from build123d import *

# Parameters (mm, degrees)
SALIENTE_EXTRUIR1_DEPTH = 35
CORTAR_EXTRUIR1_REACH   = 64.883
CROQUIS2_R              = 2.55
CROQUIS3_R              = 4.75
CORTAR_EXTRUIR2_DEPTH   = 17
CHAFL_N1_SIZE           = 15
CHAFL_N1_SIZE_2         = 21.422220101
CORTAR_EXTRUIR3_START   = -35
CROQUIS4_W              = 81
CROQUIS4_H              = 1
CORTAR_EXTRUIR3_DEPTH   = 35


with BuildPart() as part:
    # Croquis1 → Saliente-Extruir1 (new body)
    with BuildSketch(Plane(origin=(0, 0, 0), x_dir=(1, 0, 0), z_dir=(0, 1, 0))):
        with BuildLine():
            Line((22.5, 0), (40.5, 0))
            Line((40.5, 0), (40.5, -33))
            Line((40.5, -33), (-40.5, -33))
            Line((-40.5, -33), (-40.5, 0))
            Line((-40.5, 0), (-22.5, 0))
            ThreePointArc((-22.5, 0), (0, -22.5), (22.5, 0))
        make_face()
    extrude(amount=SALIENTE_EXTRUIR1_DEPTH)

    # Croquis2 → Cortar-Extruir1 (cut, up to next)
    with BuildSketch(Plane(origin=(0, 0, 0), x_dir=(-1, 0, 0), z_dir=(0, 0, -1)), mode=Mode.PRIVATE) as cortar_extruir1_sk1:
        with Locations((-31.5, 26.25)):
            Circle(CROQUIS2_R)
    cortar_extruir1_tool1 = extrude(cortar_extruir1_sk1.sketch, amount=-CORTAR_EXTRUIR1_REACH, mode=Mode.PRIVATE) & part.part
    # Croquis2 → Cortar-Extruir1 (cut, up to next)
    with BuildSketch(Plane(origin=(0, 0, 0), x_dir=(-1, 0, 0), z_dir=(0, 0, -1)), mode=Mode.PRIVATE) as cortar_extruir1_sk2:
        with Locations((-31.5, 8.75)):
            Circle(CROQUIS2_R)
    cortar_extruir1_tool2 = extrude(cortar_extruir1_sk2.sketch, amount=-CORTAR_EXTRUIR1_REACH, mode=Mode.PRIVATE) & part.part
    # Croquis2 → Cortar-Extruir1 (cut, up to next)
    with BuildSketch(Plane(origin=(0, 0, 0), x_dir=(-1, 0, 0), z_dir=(0, 0, -1)), mode=Mode.PRIVATE) as cortar_extruir1_sk3:
        with Locations((31.5, 8.75)):
            Circle(CROQUIS2_R)
    cortar_extruir1_tool3 = extrude(cortar_extruir1_sk3.sketch, amount=-CORTAR_EXTRUIR1_REACH, mode=Mode.PRIVATE) & part.part
    # Croquis2 → Cortar-Extruir1 (cut, up to next)
    with BuildSketch(Plane(origin=(0, 0, 0), x_dir=(-1, 0, 0), z_dir=(0, 0, -1)), mode=Mode.PRIVATE) as cortar_extruir1_sk4:
        with Locations((31.5, 26.25)):
            Circle(CROQUIS2_R)
    cortar_extruir1_tool4 = extrude(cortar_extruir1_sk4.sketch, amount=-CORTAR_EXTRUIR1_REACH, mode=Mode.PRIVATE) & part.part
    add(cortar_extruir1_tool1.solids().sort_by_distance((31.5, 26.25, 0))[0], mode=Mode.SUBTRACT)
    add(cortar_extruir1_tool2.solids().sort_by_distance((31.5, 8.75, 0))[0], mode=Mode.SUBTRACT)
    add(cortar_extruir1_tool3.solids().sort_by_distance((-31.5, 8.75, 0))[0], mode=Mode.SUBTRACT)
    add(cortar_extruir1_tool4.solids().sort_by_distance((-31.5, 26.25, 0))[0], mode=Mode.SUBTRACT)

    # Croquis3 → Cortar-Extruir2 (cut)
    with BuildSketch(Plane.XY.offset(33)):
        with Locations((-31.5, 26.25)):
            Circle(CROQUIS3_R)
        with Locations((-31.5, 8.75)):
            Circle(CROQUIS3_R)
        with Locations((31.5, 26.25)):
            Circle(CROQUIS3_R)
        with Locations((31.5, 8.75)):
            Circle(CROQUIS3_R)
    extrude(amount=-CORTAR_EXTRUIR2_DEPTH, mode=Mode.SUBTRACT)

    # Chaflán1
    # the kernel refuses this chamfer: 21.422220101, 15 mm, written as the material it takes off along each edge
    with BuildSketch(Plane(origin=(40.5, -55.3240023, 33), x_dir=(0.045263737714021264, 0, -0.9989750717851553), z_dir=(0, 1, 0))) as chafl_n1_piece_1:
        Polygon((CHAFL_N1_SIZE * 0.998975071785, CHAFL_N1_SIZE * 0.045263737714), (-CHAFL_N1_SIZE_2 * 0.0452637377143, CHAFL_N1_SIZE_2 * 0.998975071791), (0, 0), align=None)
    extrude(amount=145.6480046, mode=Mode.SUBTRACT)
    with BuildSketch(Plane(origin=(-40.5, -55.3240023, 33), x_dir=(0.9997533347641299, 0, 0.022209674198456895), z_dir=(0, 1, 0))) as chafl_n1_piece_2:
        Polygon((CHAFL_N1_SIZE_2 * 0.99975333477, CHAFL_N1_SIZE_2 * 0.0222096741986), (-CHAFL_N1_SIZE * 0.0222096741985, CHAFL_N1_SIZE * 0.999753334764), (0, 0), align=None)
    extrude(amount=145.6480046, mode=Mode.SUBTRACT)

    # Croquis4 → Cortar-Extruir3 (cut)
    with BuildSketch(Plane(origin=(0, 35, 0), x_dir=(1, 0, 0), z_dir=(0, 1, 0)).offset(CORTAR_EXTRUIR3_START)):
        with Locations((0, -0.5)):
            Rectangle(CROQUIS4_W, CROQUIS4_H)
    extrude(amount=CORTAR_EXTRUIR3_DEPTH, mode=Mode.SUBTRACT)


solid = part.part
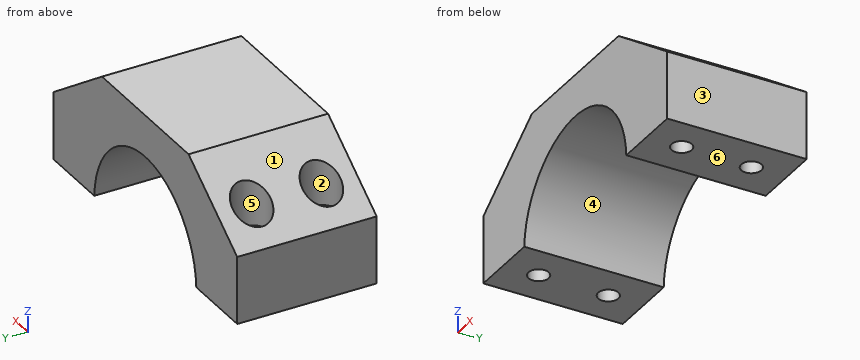
Geometry check sheet. Reference: the model listing, model coordinates, mm. Face numbers are marked on the shaded views. A direction names the side the tool comes from. Give positions to 0.01 mm unless a question says otherwise; leave off trailing zeros. Order: outer loops, then holes, each group sorted by start corner. A loop starts at its lowest first (then second) coordinate and runs counter-clockwise, first axis right, second up.
1. Sectioned sample at B-B (y = 32). Record the boundary of the cut face in (x, z), then the cut area to 3 significant figures.
Completed:
outline: (-40.5, 1) - (-22.48, 1) arc R22.5 cw to (22.48, 1) - (40.5, 1) - (40.5, 18) - (19.08, 33) - (-19.08, 33) - (-40.5, 18) - close
area: 1,520 mm2
2. Sectioned sample at A-A (z = 14). Record the boundary of the cut face in (x, y).
Completed:
outline: (-40.5, 0) - (-17.61, 0) - (-17.61, 35) - (-40.5, 35) - close; (17.61, 0) - (40.5, 0) - (40.5, 35) - (17.61, 35) - close; hole circle Ø5.1 at (-31.5, 8.75); hole circle Ø5.1 at (-31.5, 26.25); hole circle Ø5.1 at (31.5, 8.75); hole circle Ø5.1 at (31.5, 26.25)
3. Depth check by flat-ended pin: pin 1 (10.5 mm diameter, centred on x = -31.5, y = 28, fed in from +Z); pin 2 (8 mm diameter, centred on x = -31.5, y = 8.75, fed in from +Z); pin 3 (1.5 mm diameter, centred on x = 13, y = 28.5, fed in from -Z). Enter the tip coordinate at first touch or a pass-through.
Completed:
pin 1: stops at z = 27.98
pin 2: stops at z = 16
pin 3: stops at z = 17.81
4. Access from +Z, -Z, +X, -X, +Y, -Y to the whole of each face (thin tool, end or side, straight path). Record for the marked faces 1 and 2.
Completed:
face 1: +Z, -X, +Y, -Y
face 2: +Z
5. Sectioned sample at C-C (x = 31.5). Record the boundary of the cut face in (y, z), then the cut area to 3 significant figures.
Completed:
outline: (0, 1) - (6.2, 1) - (6.2, 16) - (4, 16) - (4, 24.3) - (0, 24.3) - close; (11.3, 1) - (23.7, 1) - (23.7, 16) - (21.5, 16) - (21.5, 24.3) - (13.5, 24.3) - (13.5, 16) - (11.3, 16) - close; (28.8, 1) - (35, 1) - (35, 24.3) - (31, 24.3) - (31, 16) - (28.8, 16) - close
area: 505 mm2
6. Sectioned sample at D-D (y = 8.75). Record the boundary of the cut face in (x, z).
Completed:
outline: (-40.5, 1) - (-34.05, 1) - (-34.05, 16) - (-36.25, 16) - (-36.25, 20.98) - (-40.5, 18) - close; (-28.95, 1) - (-22.48, 1) arc R22.5 cw to (22.48, 1) - (28.95, 1) - (28.95, 16) - (26.75, 16) - (26.75, 27.63) - (19.08, 33) - (-19.08, 33) - (-26.75, 27.63) - (-26.75, 16) - (-28.95, 16) - close; (34.05, 1) - (40.5, 1) - (40.5, 18) - (36.25, 20.98) - (36.25, 16) - (34.05, 16) - close
7. Scan lines: line 1 (Y direction, x = 31.5, z = 19.5); line 2 (X direction, y = 26.5, z = 8); line 3 (X direction, y = 26.5, z = 6). Record each from-to range of solid material in increasing order.
Completed:
line 1: y = 0 to 4, 13.5 to 21.5, 31 to 35
line 2: x = -40.5 to -34.04, -28.96 to -21.03, 21.03 to 28.96, 34.04 to 40.5
line 3: x = -40.5 to -34.04, -28.96 to -21.69, 21.69 to 28.96, 34.04 to 40.5
8. Draft check along X on the marked faces 3, 4, 5 and 6. Enter one of: pulls with the +X half, pulls with the -X half, needs draft (parallel to the pull), parting line crosses it, or undercut.
Completed:
face 3: pulls with the +X half
face 4: undercut
face 5: undercut
face 6: needs draft
